Can you work these out from the model? Positions are in its coordinate system, mm. A direction names the side the tool comes from. Round coordinates to 2 decimals unless told otherwise and drop trailing zeros. Write each loop counter-clockwise with the first axis right and the second up, starting at its lowest first coordinate (ties: lowest second). Pieces come first, ordered by that corner, then holes. Notation, with made-up numbers: (46.25, -6.5) - (64.25, -6.5) arc R18 ccw to (64.25, 16.5) - close; hole circle Ø3 at (86, 30.25). An arc over 180 degrees is marked (long way). One line per item, written item: value. Start each with the question number.
(1) I'm going to push flat-ended pins straight in: pin 1 Ø4 at (x, y) = (-107.5, 31.5) entering from -Z; pin 2 Ø1.5 at (y, z) = (7, 20) entering from +X; pin 3 Ø4 at (x, y) = (-22, 10) entering from +Z. Where does each tip first touch, or does it pass through?
(2) If I drill on L1, parallel to Z at x = 20, y = 21; L2, parallel to Y at x = -63, z = -21.5; L3, parallel to X at y = 32, z = 12.5, over which ranges is the centre line in solid material (lowest first)? Write a range as from..to.
(3) On a 3-axis mill with a long thin cutter (end or side, diameter ignored), from which of +Z, -Z, +X, -X, +Y, -Y can I reach the whole of each face in a straight line? I mean faces 1 (the face through (-125, 15, 0)), 2 (the face through (125, 20, 29)), 3 (the face through (21, 4, -34.5)), 4 (the face through (-127, 20, 0)), 5 (the face through (125, 20, -30)). Say none if no direction works.
(4) I want a section at A-A on z = 10. List the corners of the cut face in (x, y) for me, plus the area to 3 significant figures.
(5) I want a section at B-B on x = -51. List the corners of the cut face in (y, z) for me.
from build123d import *

# Parameters (mm, degrees)
BOSS_EXTRUDE1_DEPTH = 5
BOSS_EXTRUDE2_DEPTH = 30
SKETCH4_W           = 262
SKETCH4_H           = 45
BOSS_EXTRUDE3_DEPTH = 5


with BuildPart() as part:
    # Sketch1 → Boss-Extrude1 (new body)
    with BuildSketch(Plane(origin=(0, 0, 0), x_dir=(1, 0, 0), z_dir=(0, 1, 0))):
        Polygon((137, -22.5), (125, -22.5), (-125, -22.5), (-125, 22.5), (125, 22.5), (137, 22.5), (137, 34.5), (-137, 34.5), (-137, -34.5), (137, -34.5), align=None)
    extrude(amount=BOSS_EXTRUDE1_DEPTH)

    # Sketch2 → Boss-Extrude2 (add)
    with BuildSketch(Plane(origin=(0, 5, 0), x_dir=(1, 0, 0), z_dir=(0, 1, 0))):
        Polygon((125, 22.5), (125, 22.499356702), (137, 22.5), (137, 34.5), (125, 34.5), (125, 24.499356702), (-127, 24.499356702), (-127, -24.499356702), (125, -24.499356702), (125, -34.5), (137, -34.5), (137, -22.5), (125, -22.499356702), (125, -22.5), (-125, -22.5), (-125, 22.5), align=None)
    extrude(amount=BOSS_EXTRUDE2_DEPTH)

    # Sketch4 → Boss-Extrude3 (add)
    with BuildSketch(Plane(origin=(0, 35, 0), x_dir=(1, 0, 0), z_dir=(0, 1, 0))):
        with Locations((6, 0)):
            Rectangle(SKETCH4_W, SKETCH4_H)
    extrude(amount=-BOSS_EXTRUDE3_DEPTH)


solid = part.part
Established:
1. pin 1: z = -24.5
1. pin 2: x = -125
1. pin 3: z = 24.5
2. L1: -24.5..-22.5, 22.5..24.5
2. L2: 30..35
2. L3: -127..137
3. face 1: +X, -Y
3. face 2: +Z, -X, +Y
3. face 3: -Z, +X, -X, +Y, -Y
3. face 4: +Z, -Z, -X, +Y
3. face 5: -Z, -X, +Y
4. outline: (-137, 0) - (-125, 0) - (-125, 30) - (137, 30) - (137, 35) - (-127, 35) - (-127, 5) - (-137, 5) - close
4. area: 1,430 mm2
5. outline: (0, -34.5) - (5, -34.5) - (5, -24.5) - (35, -24.5) - (35, 24.5) - (5, 24.5) - (5, 34.5) - (0, 34.5) - (0, 22.5) - (30, 22.5) - (30, -22.5) - (0, -22.5) - close
